Input: part model. Units: mm. Frame: model coordinates. A direction names the side the tool comes from. Round coordinates to 2 decimals unless told otherwise and drop trailing zeros. Write item = value, one per line. Start each with the question number.
```python
from build123d import *

# Parameters (mm, degrees)
BOSS_EXTRUDE1_DEPTH      = 1
SKETCH2_W                = 23.3
SKETCH2_H                = 13
CUT_EXTRUDE1_DEPTH       = 3
CHAMFER1_SIZE            = 1
CHAMFER1_OF_MIRROR1_SIZE = 1
CHAMFER2_SIZE            = 1
SKETCH3_W                = 2
SKETCH3_H                = 10
BOSS_EXTRUDE2_DEPTH      = 3
SKETCH4_W                = 1
SKETCH4_H                = 10
BOSS_EXTRUDE3_DEPTH      = 2
FILLET1_R                = 0.5
FILLET1_OF_MIRROR2_R     = 0.5


with BuildPart() as part:
    # Sketch1 → Boss-Extrude1 (new body)
    with BuildSketch(Plane.XY):
        Polygon((-35, 14.75), (-35, -14.75), (-33, -16.75), (33, -16.75), (35, -14.75), (35, 14.75), (33, 16.75), (-33, 16.75), align=None)
    extrude(amount=BOSS_EXTRUDE1_DEPTH)

    # Sketch2 → Cut-Extrude1 (cut)
    with BuildSketch(Plane.XY.offset(1)):
        with Locations((-14.5, -1.75)):
            Rectangle(SKETCH2_W, SKETCH2_H)
    cut_extrude1 = extrude(amount=-CUT_EXTRUDE1_DEPTH, mode=Mode.SUBTRACT)

    # Chamfer1
    chamfer1_edges = [part.edges().sort_by_distance(p)[0] for p in [
        (-14.5, -8.25, 1),
        (-2.85, -1.75, 1),
        (-14.5, 4.75, 1),
        (-26.15, -1.75, 1),
    ]]
    chamfer(chamfer1_edges, length=CHAMFER1_SIZE - 0.0001)  # a hair under: the kernel refuses the full size

    # Mirror1: Cut-Extrude1 across plane
    add(cut_extrude1.mirror(Plane(origin=(0, 0, 0), x_dir=(0, 0, 1), z_dir=(1, 0, 0))), mode=Mode.SUBTRACT)

    # Chamfer1 of Mirror1
    chamfer1_of_mirror1_edges = [part.edges().sort_by_distance(p)[0] for p in [
        (14.5, -8.25, 1),
        (2.85, -1.75, 1),
        (14.5, 4.75, 1),
        (26.15, -1.75, 1),
    ]]
    chamfer(chamfer1_of_mirror1_edges, length=CHAMFER1_OF_MIRROR1_SIZE - 0.0001)  # a hair under: the kernel refuses the full size

    # Chamfer2
    chamfer2_edges = [part.edges().sort_by_distance(p)[0] for p in [
        (35, 0, 1),
        (34, 15.75, 1),
        (0, 16.75, 1),
        (-34, 15.75, 1),
        (-35, 0, 1),
        (34, -15.75, 1),
        (0, -16.75, 1),
        (-34, -15.75, 1),
    ]]
    chamfer(chamfer2_edges, length=CHAMFER2_SIZE - 0.0001)  # a hair under: the kernel refuses the full size

    # Sketch3 → Boss-Extrude2 (add)
    with BuildSketch(Plane(origin=(0, 0, 0), x_dir=(-1, 0, 0), z_dir=(0, 0, -1))):
        with Locations((-31.5, 0)):
            Rectangle(SKETCH3_W, SKETCH3_H)
    boss_extrude2 = extrude(amount=BOSS_EXTRUDE2_DEPTH)

    # Sketch4 → Boss-Extrude3 (add)
    with BuildSketch(Plane(origin=(32.5, 0, 0), x_dir=(0, 0, -1), z_dir=(1, 0, 0))):
        with Locations((2.5, 0)):
            Rectangle(SKETCH4_W, SKETCH4_H)
    boss_extrude3 = extrude(amount=BOSS_EXTRUDE3_DEPTH)

    # Fillet1
    fillet1_edges = [part.edges().sort_by_distance(p)[0] for p in [
        (34.5, 0, -3),
        (34.5, 5, -2.5),
        (34.5, 0, -2),
        (34.5, -5, -2.5),
    ]]
    fillet(fillet1_edges, radius=FILLET1_R - 0.0001)  # a hair under: the kernel refuses the full size

    # Mirror2: Boss-Extrude2, Boss-Extrude3 across plane
    add(boss_extrude2.mirror(Plane(origin=(0, 0, 0), x_dir=(0, 0, 1), z_dir=(1, 0, 0))))
    add(boss_extrude3.mirror(Plane(origin=(0, 0, 0), x_dir=(0, 0, 1), z_dir=(1, 0, 0))))

    # Fillet1 of Mirror2
    fillet1_of_mirror2_edges = [part.edges().sort_by_distance(p)[0] for p in [
        (-34.5, 0, -3),
        (-34.5, 5, -2.5),
        (-34.5, 0, -2),
        (-34.5, -5, -2.5),
    ]]
    fillet(fillet1_of_mirror2_edges, radius=FILLET1_OF_MIRROR2_R - 0.0001)  # a hair under: the kernel refuses the full size

    # Chamfer3: read off the stored shape, not the designer's step
    # Chamfer3: loft between two sections, ruled curve by curve
    chamfer3_from = [
        Edge.make_line((32.5, -5, -3), (30.5, -5, -3)),
        Edge.make_line((30.5, -5, -3), (30.5, 5, -3)),
        Edge.make_line((30.5, 5, -3), (32.5, 5, -3)),
        Edge.make_line((32.5, 5, -3), (32.5, -5, -3)),
    ]
    chamfer3_to = [
        Edge.make_line((32.5, -7, 0), (28.5, -7, 0)),
        Edge.make_line((28.5, -7, 0), (28.5, 7, 0)),
        Edge.make_line((28.5, 7, 0), (32.5, 7, 0)),
        Edge.make_line((32.5, 7, 0), (32.5, -7, 0)),
    ]
    chamfer3 = Solid(Shell([*[Face.make_surface_from_curves(chamfer3_from[k], chamfer3_to[k]) for k in range(4)], Face(Wire(chamfer3_from)), Face(Wire(chamfer3_to))]))
    add(chamfer3)

    # Chamfer4: read off the stored shape, not the designer's step
    # Chamfer4: loft between two sections, ruled curve by curve
    chamfer4_from = [
        Edge.make_line((-32.5, -5, -3), (-30.5, -5, -3)),
        Edge.make_line((-32.5, 5, -3), (-30.5, 5, -3)),
        Edge.make_line((-30.5, 5, -3), (-30.5, -5, -3)),
        Edge.make_line((-32.5, 5, -3), (-32.5, -5, -3)),
    ]
    chamfer4_to = [
        Edge.make_line((-32.5, -7, 0), (-28.5, -7, 0)),
        Edge.make_line((-32.5, 7, 0), (-28.5, 7, 0)),
        Edge.make_line((-28.5, 7, 0), (-28.5, -7, 0)),
        Edge.make_line((-32.5, 7, 0), (-32.5, -7, 0)),
    ]
    chamfer4 = Solid(Shell([*[Face.make_surface_from_curves(chamfer4_from[k], chamfer4_to[k]) for k in range(4)], Face(Wire(chamfer4_from)), Face(Wire(chamfer4_to))]))
    add(chamfer4)


solid = part.part
```
1. Section B-B (y = 0.5). State how many separate pieces and enclosed holes the cut face has, then the cut area to 3 significant figures.
2. Line query: line 1 along Z through (x, y) = (14.5, 12.5); line 2 along Y through (x, z) = (10.5, 0.55); line 3 along Y through (x, z) = (5.5, 0.5). Output: solid intervals per line, ascending.
3. Reachability of faces 4 (the flat face through (33, 0, -2)), 5 (the flat face through (0, 0, 1)), 6 (the flat face through (-33, 0, -2)) from +Z, -Z, +X, -X, +Y, -Y: full face, straight path, thin tool, end or side. Return the list, or none.
4. Pin query (flat end, axial travel): P1, Ø2, axis at y = 3, z = -1.5, coming from the -X side; P2, Ø6, axis at x = -18, y = -3.5, coming from the -Z side; P3, Ø10, axis at x = 12.5, y = -8.5, coming from the -Z side; P4, Ø0.8, axis at x = 33.5, z = -2.5, coming from the -Y side. Return the tip coordinate at first contact, or that it passes through.
5. Mould query, pull axis X, two halves, no side actions, for faces 1 (the flat face through (33.67, 15.39, 0.49)), 2 (the flat face through (32, 0, -3)), 3 (the flat face through (-33.64, 15.42, 0.49)). Classes: pulls with the +X half, pulls with the -X half, needs draft (parallel to the pull), parting line crosses it, or undercut.
Check sheet entries:
q1.separate_pieces = 3
q1.enclosed_holes = 0
q1.area = 42.2 mm2
q2.line_1 = 0 to 1
q2.line_2 = -16.2 to -8.8, 5.3 to 16.2
q2.line_3 = -16.25 to -8.75, 5.25 to 16.25
q3.face_4 = +X, +Y, -Y
q3.face_5 = +Z, +X, -X, +Y, -Y
q3.face_6 = -X, +Y, -Y
q4.P1 = -34.5
q4.P2 = through
q4.P3 = 0
q4.P4 = -5
q5.face_1 = pulls with the +X half
q5.face_2 = needs draft
q5.face_3 = pulls with the -X half
